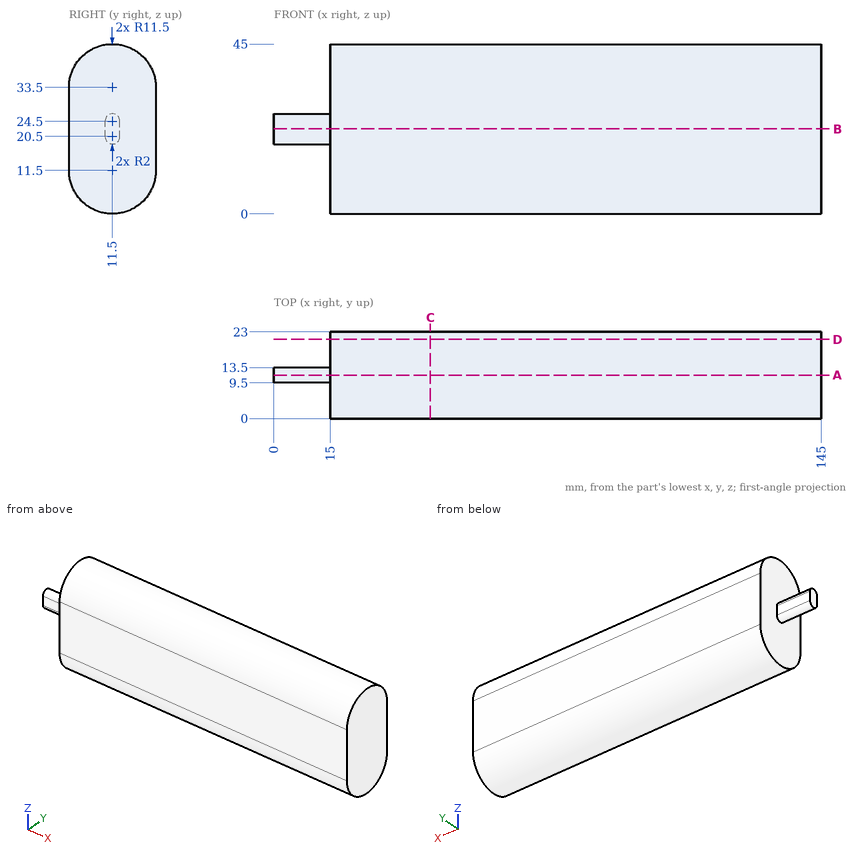
Input: dimensioned drawing with shaded views. Units: mm. Origin: part minimum x, y, z. Round coordinates to 2 decimals unless told otherwise and drop trailing zeros. Order: outer loops, then holes, each group sorted by start corner. A loop starts at its lowest first (then second) coordinate and runs counter-clockwise, first axis right, second up. Notation, with made-up numbers: M -39.5,68.5 L 11.5,68.5 A30 ccw 11.5,92.5 Z; hole C 47.5,84.25 d10. An arc over 180 degrees is marked long. Use one line per item in the form item = value. Start each with the question number.
Q1. Pin query (flat end, axial travel): pin 1 Ø3 at (x, y) = (82.5, 13.5) entering from +Z; pin 2 Ø5 at (x, y) = (58, 17.5) entering from +Z; pin 3 Ø1.5 at (y, z) = (7, 27) entering from -X. Return the tip coordinate at first contact, or that it passes through.
Q2. Cut plane B-B (z = 22.5). Return loops of the section in (x, y).
Q3. Cut plane C-C (x = 41.5). Return loops of the section in (y, z).
Q4. Cut plane A-A (y = 11.5). Return loops of the section in (x, z), and give its area (3 significant figures).
Q5. Cut plane D-D (y = 21). Return loops of the section in (x, z).
Q6. Material intervals for line 1 (X direction, y = 16, z = 43); line 2 (Y direction, x = 114, z = 34); line 3 (Y direction, x = 138.5, z = 37.5), sorted ascending. Write a range as [from, to].
Geometry results:
q1.pin_1 = 44.99
q1.pin_2 = 44.45
q1.pin_3 = 15
q2.outline = M 0,9.5 L 15,9.5 L 15,0 L 145,0 L 145,23 L 15,23 L 15,13.5 L 0,13.5 Z
q3.outline = M 0,11.5 A11.5 ccw 23,11.5 L 23,33.5 A11.5 ccw 0,33.5 Z
q4.outline = M 0,18.5 L 15,18.5 L 15,0 L 145,0 L 145,45 L 15,45 L 15,26.5 L 0,26.5 Z
q4.area = 5,970 mm^2
q5.outline = M 15,5.02 L 145,5.02 L 145,39.98 L 15,39.98 Z
q6.line_1 = [15, 145]
q6.line_2 = [0.01, 22.99]
q6.line_3 = [0.72, 22.28]
